Model file for the job. Use its own axes, mm. A direction names the side the tool comes from. Coordinates: 2 decimals unless noted, no trailing zeros. Order: outer loops, then holes, each group sorted by start corner. A loop starts at its lowest first (then second) coordinate and runs counter-clockwise, first axis right, second up.
from build123d import *

# Parameters (mm, degrees)
SKETCH1_W           = 155
SKETCH1_H           = 155
SKETCH1_R           = 3
SKETCH1_R_2         = 60
BOSS_EXTRUDE1_DEPTH = 1
FILLET1_R           = 3
SKETCH2_R           = 65
SKETCH2_R_2         = 60
BOSS_EXTRUDE2_DEPTH = 7


with BuildPart() as part:
    # Sketch1 → Boss-Extrude1 (new body)
    with BuildSketch(Plane(origin=(0, 0, 0), x_dir=(1, 0, 0), z_dir=(0, 1, 0))):
        Rectangle(SKETCH1_W, SKETCH1_H)
        with Locations((-68, 69.5)):
            Circle(SKETCH1_R, mode=Mode.SUBTRACT)
        with Locations((68, 69.5)):
            Circle(SKETCH1_R, mode=Mode.SUBTRACT)
        with Locations((-68, -69.5)):
            Circle(SKETCH1_R, mode=Mode.SUBTRACT)
        with Locations((68, -69.5)):
            Circle(SKETCH1_R, mode=Mode.SUBTRACT)
        Circle(SKETCH1_R_2, mode=Mode.SUBTRACT)
    extrude(amount=BOSS_EXTRUDE1_DEPTH)

    # Fillet1
    fillet1_edges = [part.edges().sort_by_distance(p)[0] for p in [
        (77.5, 0.5, 77.5),
        (-77.5, 0.5, 77.5),
        (-77.5, 0.5, -77.5),
        (77.5, 0.5, -77.5),
    ]]
    fillet(fillet1_edges, radius=FILLET1_R)

    # Sketch2 → Boss-Extrude2 (add)
    with BuildSketch(Plane(origin=(0, 1, 0), x_dir=(1, 0, 0), z_dir=(0, 1, 0))):
        Circle(SKETCH2_R)
        Circle(SKETCH2_R_2, mode=Mode.SUBTRACT)
    extrude(amount=-BOSS_EXTRUDE2_DEPTH)


solid = part.part
Q1. Drop flat-ended pins along their axis: P1, Ø7, axis at x = 68, z = -69.5, coming from the +Y side; P2, Ø4, axis at y = -5, z = 9.5, coming from the -X side; P3, Ø1.5, axis at x = -55.5, y = -4, coming from the -Z side. Give the stop position or say it passes through.
Established:
P1: stops at y = 1
P2: stops at x = -64.57
P3: stops at z = -35.03
Q2. Probe line 1 (Z direction, x = -68, y = 0.5); line 2 (X direction, y = 0.45, z = 69.5); line 3 (X direction, y = 0.2, z = 0). List the from-to ranges inside material, lowest first.
Established:
line 1: z = -77.5 to -72.5, -66.5 to 66.5, 72.5 to 77.5
line 2: x = -77.5 to -71, -65 to 65, 71 to 77.5
line 3: x = -77.5 to -60, 60 to 77.5
Q3. Cut at B-B, the plane x = 68. List the corners of the cut face in (y, z).
Established:
outline: (0, -77.5) - (1, -77.5) - (1, -72.5) - (0, -72.5) - close; (0, -66.5) - (1, -66.5) - (1, 66.5) - (0, 66.5) - close; (0, 72.5) - (1, 72.5) - (1, 77.5) - (0, 77.5) - close
Q4. Mould opens along X. For faces 3 (the face through (19, -6, 57.5)), 4 (the face through (-70.4, 0.5, 71.3)), 5 (the face through (-70.4, 0.5, -67.7)), 6 (the face through (62, -2.96, -19.52)) say: pulls with the +X half, pulls with the -X half, needs draft (parallel to the pull), parting line crosses it, or undercut.
Established:
face 3: needs draft
face 4: undercut
face 5: undercut
face 6: parting line crosses it
Q5. Which spindle directions (+Z, -Z, +X, -X, +Y, -Y) get a long thin tool onto all of the face, cutting with end or side? Do faces 1 (the face through (65.6, 0.5, -67.7)), 2 (the face through (-70, 0, -1)). Say none if no direction does.
Established:
face 1: +Y, -Y
face 2: -Y
Q6. Cut at D-D, the plane z = 0. List the corners of the cut face in (x, y).
Established:
outline: (-77.5, 0) - (-65, 0) - (-65, -6) - (-60, -6) - (-60, 1) - (-77.5, 1) - close; (60, -6) - (65, -6) - (65, 0) - (77.5, 0) - (77.5, 1) - (60, 1) - close
Q7. Cut at C-C, the plane x = 0. List the corners of the cut face in (y, z), plus the area to 3 significant figures.
Established:
outline: (-6, -65) - (0, -65) - (0, -77.5) - (1, -77.5) - (1, -60) - (-6, -60) - close; (-6, 60) - (1, 60) - (1, 77.5) - (0, 77.5) - (0, 65) - (-6, 65) - close
area: 95.0 mm2
Q8. Cut at A-A, the plane z = 69.5. List the corners of the cut face in (x, y), plus the area to 3 significant figures.
Established:
outline: (-77.5, 0) - (-71, 0) - (-71, 1) - (-77.5, 1) - close; (-65, 0) - (65, 0) - (65, 1) - (-65, 1) - close; (71, 0) - (77.5, 0) - (77.5, 1) - (71, 1) - close
area: 143 mm2
